from build123d import *

# Parameters (mm, degrees)
SKETCH2_W           = 76.2
SKETCH2_H           = 76.2
BOSS_EXTRUDE1_DEPTH = 76.2
SKETCH3_R           = 4.7625
SKETCH3_R_2         = 5.5626
CUT_EXTRUDE1_DEPTH  = 72.39
SKETCH5_R           = 5.5626
BOSS_EXTRUDE2_DEPTH = 62.23


with BuildPart() as part:
    # Sketch2 → Boss-Extrude1 (new body)
    with BuildSketch(Plane(origin=(0, 0, 0), x_dir=(1, 0, 0), z_dir=(0, 1, 0))):
        Rectangle(SKETCH2_W, SKETCH2_H)
    extrude(amount=BOSS_EXTRUDE1_DEPTH)

    # Sketch3 → Cut-Extrude1 (cut)
    with BuildSketch(Plane.XY.offset(38.1)):
        with Locations((0, 26.522528218)):
            Circle(SKETCH3_R)
        with Locations((0, 52.367028218)):
            Circle(SKETCH3_R_2)
    extrude(amount=-CUT_EXTRUDE1_DEPTH, mode=Mode.SUBTRACT)

    # Sketch5 → Boss-Extrude2 (add)
    with BuildSketch(Plane.XY.offset(-34.29)):
        with Locations((0, 52.367028218)):
            Circle(SKETCH5_R)
    extrude(amount=BOSS_EXTRUDE2_DEPTH)


solid = part.part
Can you work these out from the model? Positions are in its coordinate system, mm. A direction names the side the tool comes from. Give positions to 0.01 mm unless a question says otherwise; leave off trailing zeros. Order: outer loops, then holes, each group sorted by start corner. A loop starts at its lowest first (then second) coordinate and runs counter-clockwise, first axis right, second up. Notation, with made-up numbers: M 37.25,36.25 L 46.25,36.25 A22 cw 46.25,61.25 Z; hole C 12.5,-15.5 d3. An arc over 180 degrees is marked long. Use a Markdown table: item, result. Add a question column.
Item 1: We'd pull the mould along Y, two halves only. Please class faces 1 (the flat face through (-1, 0, -1)), 2 (the flat face through (-1, 38, -38.1)), 3 (the flat face through (0, 27, -34.29)): +Y half, -Y half, draft (parallel to the pull), parting line (faces both ways), or undercut.
Item 2: Suppose I cut it at C-C (y = 25). List the corners of the cut face in (x, z) for me, then the cut area to 3 significant figures.
Item 3: Suppose I cut it at B-B (y = 49.5). List the corners of the cut face in (x, z) for me, then the cut area to 3 significant figures.
Item 4: Will these pins go through, and if not, where does the flat tip stop? pin 1 (6.5 mm diameter, centred on x = 0, y = 52.37, fed in from +Z); pin 2 (3 mm diameter, centred on x = 2, y = 24.5, fed in from +Z).
Item 5: Suppose I cut it at A-A (x = 0). List the corners of the cut face in (y, z) for me, then the cut area to 3 significant figures.
Item 6: If I drill on L1, parallel to Y at x = 0, z = 30.5; L2, parallel to Y at x = 0, z = 7, over which ranges is the centre line in solid material (lowest first)? Write a range as [from, to].
Item 7: For faces 4 (the cylindrical face through (-1.206, 46.937, 33.091)), 5 (the flat face through (-38.1, 38, 1)), which set-ups out of +Z, -Z, +X, -X, +Y, -Y let a thin tool reach every point of the face, with its end or its side?
Answer sheet:
| question | item | result |
|---|---|---|
| 1 | face 1 | -Y half |
| 1 | face 2 | draft |
| 1 | face 3 | undercut |
| 2 | outline | M -38.1,-38.1 L 38.1,-38.1 L 38.1,38.1 L 4.51,38.1 L 4.51,-34.29 L -4.51,-34.29 L -4.51,38.1 L -38.1,38.1 Z |
| 2 | area | 5,150 mm² |
| 3 | outline | M -38.1,-38.1 L 38.1,-38.1 L 38.1,38.1 L 4.77,38.1 L 4.77,27.94 L -4.77,27.94 L -4.77,38.1 L -38.1,38.1 Z |
| 3 | area | 5,710 mm² |
| 4 | pin 1 | stops at z = 27.94 |
| 4 | pin 2 | stops at z = -34.29 |
| 5 | outline | M 0,-38.1 L 76.2,-38.1 L 76.2,38.1 L 57.93,38.1 L 57.93,27.94 L 46.8,27.94 L 46.8,38.1 L 31.29,38.1 L 31.29,-34.29 L 21.76,-34.29 L 21.76,38.1 L 0,38.1 Z |
| 5 | area | 5,000 mm² |
| 6 | L1 | y = [0, 21.76], [31.29, 46.8], [57.93, 76.2] |
| 6 | L2 | y = [0, 21.76], [31.29, 76.2] |
| 7 | face 4 | +Z |
| 7 | face 5 | +Z, -Z, -X, +Y, -Y |
